from build123d import *

# Parameters (mm, degrees)
BOSS_EXTRUDE1_DEPTH = 1.6
SKETCH2_W           = 30
SKETCH2_H           = 5
BOSS_EXTRUDE2_DEPTH = 1.15
SKETCH3_R           = 4.1
BOSS_EXTRUDE3_DEPTH = 10.5


with BuildPart() as part:
    # Sketch1 → Boss-Extrude1 (new body)
    with BuildSketch(Plane(origin=(0, 0, 0), x_dir=(1, 0, 0), z_dir=(0, 1, 0))):
        Polygon((-18, 26.5), (-18, -19.25), (-10.75, -26.5), (10.75, -26.5), (18, -19.25), (18, 26.5), align=None)
    extrude(amount=BOSS_EXTRUDE1_DEPTH)

    # Sketch2 → Boss-Extrude2 (add)
    with BuildSketch(Plane.XZ):
        with Locations((0, -14.7)):
            Rectangle(SKETCH2_W, SKETCH2_H)
    extrude(amount=BOSS_EXTRUDE2_DEPTH)

    # Sketch3 → Boss-Extrude3 (add)
    with BuildSketch(Plane(origin=(0, 1.6, 0), x_dir=(1, 0, 0), z_dir=(0, 1, 0))):
        with Locations((-9.25, 21.3)):
            Circle(SKETCH3_R)
        with Locations((3.5, 21.3)):
            Circle(SKETCH3_R)
    extrude(amount=BOSS_EXTRUDE3_DEPTH)


solid = part.part
Here's how the part is built. I have some questions about the finished solid (model axes, mm). A direction names the side the tool comes from. Coordinates: 2 decimals unless noted, no trailing zeros. Order: outer loops, then holes, each group sorted by start corner. A loop starts at its lowest first (then second) coordinate and runs counter-clockwise, first axis right, second up. Notation, with made-up numbers: (14, 4.25) - (26, 4.25) arc R32 ccw to (26, 38.25) - close; hole circle Ø7 at (31.5, -36). An arc over 180 degrees is marked (long way). Use CSV: the item, a comma, the result in double quotes. Start each with the question number.
1. Please list where these lines run through material, in increasing order: line 1 (Y direction, x = 4.5, z = 22); line 2 (Z direction, x = -14.5, y = -0.25); line 3 (Z direction, x = -9.5, y = 11). Write a range as from..to.
2. If we mould it in two halves opening along X, with no side actions, what happens to faces 1 (the face through (-18, 1, -4)), 2 (the face through (-12.5, 6.8, -18.8)), 3 (the face through (0, 1, -26.5))? For each: +X half, -X half, draft (parallel to the pull), parting line (faces both ways), or undercut.
3. For faces 4 (the face through (5.39, 6.78, -17.66)), 5 (the face through (15, -0.6, -14.7)), 6 (the face through (-0.2, -0.6, -12.2)), 7 (the face through (-0.2, -0.6, -17.2)), 8 (the face through (-15, -0.6, -14.7)), which set-ups out of +Z, -Z, +X, -X, +Y, -Y let a thin tool reach every point of the face, with its end or its side?
4. Suppose I cut it at B-B on z = -21.3. List the corners of the cut face in (x, y) for me, then the cut area to 3 significant figures.
5. Suppose I cut it at A-A on x = 3.5. List the corners of the cut face in (y, z) for me, then the cut area to 3 significant figures.
6. Suppose I cut it at C-C on y = 5.75. List the corners of the cut face in (x, z) for me.
7. Suppose I cut it at D-D on z = 20. List the corners of the cut face in (x, y) for me.
8. I'm going to push flat-ended pins straight in: pin 1 (1.3 mm diameter, centred on x = -5.5, y = -0.5, fed in from +Z); pin 2 (6 mm diameter, centred on x = 5.5, z = 10.5, fed in from +Y); pin 3 (1.5 mm diameter, centred on x = 3.5, z = -3, fed in from -Y); pin 4 (1.5 mm diameter, centred on x = 9.5, y = 6.5, fed in from +Z). Where does each tip first touch, or does it pass through?
Output:
1,line 1,"y = 0..1.6"
1,line 2,"z = -17.2..-12.2"
1,line 3,"z = -25.39..-17.21"
2,face 1,"-X half"
2,face 2,"undercut"
2,face 3,"draft"
3,face 4,"+Y"
3,face 5,"+Z, -Z, +X, -Y"
3,face 6,"+Z, +X, -X, -Y"
3,face 7,"-Z, +X, -X, -Y"
3,face 8,"+Z, -Z, -X, -Y"
4,outline,"(-18, 0) - (18, 0) - (18, 1.6) - (7.6, 1.6) - (7.6, 12.1) - (-0.6, 12.1) - (-0.6, 1.6) - (-5.15, 1.6) - (-5.15, 12.1) - (-13.35, 12.1) - (-13.35, 1.6) - (-18, 1.6) - close"
4,area,"230 mm2"
5,outline,"(-1.15, -17.2) - (0, -17.2) - (0, -26.5) - (1.6, -26.5) - (1.6, -25.4) - (12.1, -25.4) - (12.1, -17.2) - (1.6, -17.2) - (1.6, 26.5) - (0, 26.5) - (0, -12.2) - (-1.15, -12.2) - close"
5,area,"177 mm2"
6,outline,"circle Ø8.2 at (-9.25, -21.3); circle Ø8.2 at (3.5, -21.3)"
7,outline,"(-17.25, 0) - (17.25, 0) - (17.25, 1.6) - (-17.25, 1.6) - close"
8,pin 1,"stops at z = 26.5"
8,pin 2,"stops at y = 1.6"
8,pin 3,"stops at y = 0"
8,pin 4,"passes through"
